```python
from build123d import *

# Parameters (mm, degrees)
F0_R     = 12.5
F0_R_2   = 5
F1_DEPTH = 10
F3_DEPTH = 7.5
F5_DEPTH = 2
F6_W     = 5
F6_H     = 7.917322
F7_DEPTH = 2


with BuildPart() as f1:
    # F0 (on Top) → F1 (new body)
    with BuildSketch(Plane.XY):
        Circle(F0_R)
        Circle(F0_R_2, mode=Mode.SUBTRACT)
    extrude(amount=F1_DEPTH)

    # F2 (on face) → F3 (cut, symmetric)
    with BuildSketch(Plane.XY.offset(10)):
        with BuildLine():
            Line((-2.5, -4.330127), (-2.5, -12.247449))
            ThreePointArc((-2.5, -12.247449), (0, -12.5), (2.5, -12.247449))
            Line((2.5, -12.247449), (2.5, -4.330127))
            ThreePointArc((2.5, -4.330127), (0, -5), (-2.5, -4.330127))
        make_face()
        with BuildLine():
            ThreePointArc((2.5, 12.247449), (0, 12.5), (-2.5, 12.247449))
            Line((-2.5, 12.247449), (-2.5, 4.330127))
            ThreePointArc((-2.5, 4.330127), (0, 5), (2.5, 4.330127))
            Line((2.5, 4.330127), (2.5, 12.247449))
        make_face()
    extrude(amount=F3_DEPTH, both=True, mode=Mode.SUBTRACT)

    # F4 (on face) → F5 (join)
    with BuildSketch(Plane.XY.offset(10)):
        Polygon((-2.5, -4.330127), (-2.5, -12.247449), (2.568516, -12.247449), (2.568516, -4.281065), align=None)
    extrude(amount=-F5_DEPTH)

    # F6 (on face) → F7 (join)
    with BuildSketch(Plane.XY.offset(10)):
        with Locations((0, 8.288788)):
            Rectangle(F6_W, F6_H)
    extrude(amount=-F7_DEPTH)


solid = f1.part
```
Can you work these out from the model? Positions are in its coordinate system, mm. A direction names the side the tool comes from. Give positions to 0.01 mm unless a question says otherwise; leave off trailing zeros. Write each loop counter-clockwise with the first axis right and the second up, starting at its lowest first coordinate (ties: lowest second). Pieces come first, ordered by that corner, then holes. Notation, with made-up numbers: (-4.75, 26) -> (7.25, 26) arc R23 ccw to (7.25, 53) -> close; hole circle Ø9 at (38, 28). An arc over 180 degrees is marked (long way). One line per item, written item: value.
Q1. Imagine slicing it at A-A on y = 0. Please give me the cut outline in (x, z).
Results found:
outline: (-12.5, 0) -> (-5, 0) -> (-5, 10) -> (-12.5, 10) -> close; (5, 0) -> (12.5, 0) -> (12.5, 10) -> (5, 10) -> close
Q2. Please list where these lines run through material, in increasing order: line 1 (X direction, y = 1, z = 2.25); line 2 (Z direction, x = -1, y = 5.5); line 3 (X direction, y = -4, z = 1.25). Write a range as [from, to].
Results found:
line 1: x = [-12.46, -4.9], [4.9, 12.46]
line 2: z = [0, 2.5], [8, 10]
line 3: x = [-11.84, -3], [3, 11.84]
Q3. For P1, Ø1.6, axis at y = 7, z = 5, coming from the -X side; P2, Ø1.6, axis at x = 0.5, z = 9.5, coming from the -Y side; P3, Ø2, axis at x = -0.5, z = 8.5, coming from the +Y side, each with a flat end and sliding along its axis, tell me the tip position at first contact or that it passes through.
Results found:
P1: stops at x = -10.85
P2: stops at y = -12.25
P3: stops at y = 12.25
Q4. Imagine slicing it at C-C on x = 0. Please give me the cut outline in (y, z), and give its area (3 significant figures).
Results found:
outline: (-12.5, 0) -> (-5, 0) -> (-5, 2.5) -> (-12.5, 2.5) -> close; (-12.25, 8) -> (-4.31, 8) -> (-4.31, 10) -> (-12.25, 10) -> close; (4.33, 8) -> (12.25, 8) -> (12.25, 10) -> (4.33, 10) -> close; (5, 0) -> (12.5, 0) -> (12.5, 2.5) -> (5, 2.5) -> close
area: 69.2 mm^2
Q5. Which directions (+Z, -Z, +X, -X, +Y, -Y) give clear straight access to the entire face, cutting with the end or side of a thin tool? Please do faces 1 (the face through (0, 12.247, 9)), 2 (the face through (-2.5, -8, 5)), 3 (the face through (5.77, -11.09, 4.93)).
Results found:
face 1: +Z, +X, -X, +Y
face 2: +Y, -Y
face 3: +Z, -Z
Q6. Imagine slicing it at B-B on z = 5.5. Please give me the cut outline in (x, y).
Results found:
outline: (-2.5, -12.25) -> (-2.5, -4.33) arc R5 cw to (-2.5, 4.33) -> (-2.5, 12.25) arc R12.5 ccw to start; (2.5, -12.25) arc R12.5 ccw to (2.5, 12.25) -> (2.5, 4.33) arc R5 cw to (2.5, -4.33) -> close
Q7. We'd pull the mould along Y, two halves only. Please class faces 4 (the face through (0, -12.247, 9)), 5 (the face through (2.5, -8, 5)), 6 (the face through (0, 4.33, 9)): +Y half, -Y half, draft (parallel to the pull), parting line (faces both ways), or undercut.
Results found:
face 4: -Y half
face 5: draft
face 6: undercut
Q8. Imagine slicing it at D-D on y = 11.25. Please give me the cut outline in (x, z), and give its area (3 significant figures).
Results found:
outline: (-5.45, 0) -> (5.45, 0) -> (5.45, 10) -> (-5.45, 10) -> close; hole (-2.5, 2.5) -> (2.5, 2.5) -> (2.5, 8) -> (-2.5, 8) -> close
area: 81.5 mm^2
